from build123d import *

# Parameters (mm, degrees)
BOSS_EXTRUDE1_DEPTH = 6
FILLET2_R           = 20
SKETCH7_R           = 4
CUT_EXTRUDE3_DEPTH  = 5


with BuildPart() as part:
    # Sketch4 → Boss-Extrude1 (new body)
    with BuildSketch(Plane(origin=(0, 0, 0), x_dir=(1, 0, 0), z_dir=(0, 1, 0))):
        Polygon((-87.5, -50), (87.5, -50), (87.5, 0), (87.5, 60.006143386), (-87.5, 0), align=None)
    extrude(amount=BOSS_EXTRUDE1_DEPTH)

    # Fillet2
    fillet2_edges = [part.edges().sort_by_distance(p)[0] for p in [
        (87.5, 3, -60.006143386),
    ]]
    fillet(fillet2_edges, radius=FILLET2_R)

    # Sketch7 → Cut-Extrude3 (cut)
    with BuildSketch(Plane(origin=(0, 6, 0), x_dir=(1, 0, 0), z_dir=(0, 1, 0))):
        with Locations(Location((62.5, 25, 0), (0, 0, 270))):
            Circle(SKETCH7_R)
    extrude(amount=-CUT_EXTRUDE3_DEPTH, mode=Mode.SUBTRACT)


solid = part.part
Geometry check sheet. Reference: the model listing, model coordinates, mm. Round coordinates to 2 decimals unless told otherwise and drop trailing zeros. Loops run counter-clockwise (first coordinate to the right, second up) from the corner with the lowest first, then second, coordinate; pieces in that order, holes last. Notation, with made-up numbers: (61, 20.5) - (66, 20.5) arc R12 ccw to (66, 38.5) - close; hole circle Ø1 at (1, 84.25). An arc over 180 degrees is marked (long way). One line per question, with ' | ' between items. Start each with the question number.
1. Cross-section at C-C on x = 76. Record the cut outline in (y, z), then the cut area to 3 significant figures.
2. Cross-section at B-B on z = -25. Record the cut outline in (x, y).
3. Depth check by flat-ended pin: pin 1 (1.5 mm diameter, centred on x = 69.5, y = 4.5, fed in from -Z). Enter the tip coordinate at first touch or a pass-through.
4. Cross-section at A-A on y = 2.55. Record the cut outline in (x, z), then the cut area to 3 significant figures.
5. Draft check along X on faces 1 (the face through (-12.2, 2.96, -25.82)), 2 (the face through (63, 1, -25)), 3 (the face through (79.34, 3.042, -48.124)), 4 (the face through (58.595, 3.535, -25.867)). Enter one of: released by +X, released by -X, zero draft, split by the parting line, or undercut.
6. Cross-section at D-D on z = -36. Record the cut outline in (x, y), then the cut area to 3 significant figures.
7. Scan lines: line 1 (Z direction, x = 72, y = 1.2); line 2 (Z direction, x = 50, y = 4.05). Record each from-to range of solid material in increasing order. Write a range as [from, to].
Taken from the geometry:
1) outline: (0, -50.11) - (6, -50.11) - (6, 50) - (0, 50) - close | area: 601 mm²
2) outline: (-14.59, 0) - (87.5, 0) - (87.5, 6) - (66.5, 6) - (66.5, 1) - (58.5, 1) - (58.5, 6) - (-14.59, 6) - close
3) pin 1: z = -51.97
4) outline: (-87.5, 0) - (61.01, -50.92) arc R20 ccw to (87.5, -32.01) - (87.5, 50) - (-87.5, 50) - close; hole circle Ø8 at (62.5, -25) | area: 13,800 mm²
5) face 1: released by -X | face 2: undercut | face 3: split by the parting line | face 4: undercut
6) outline: (17.49, 0) - (87.1, 0) - (87.1, 6) - (17.49, 6) - close | area: 418 mm²
7) line 1: [-51.49, 50] | line 2: [-47.15, 50]
